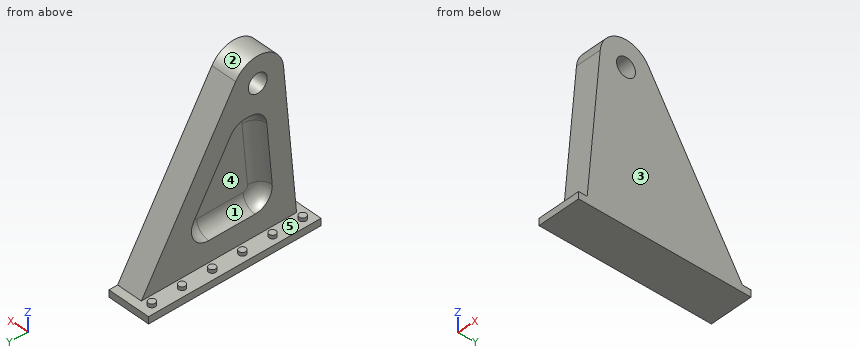
from build123d import *

# Parameters (mm, degrees)
F0_W          = 20
F0_H          = 0.8
F1_DEPTH      = 3
F1_DEPTH_BACK = 2
F2_R          = 1.1
F3_DEPTH      = 3
F5_DEPTH      = 1.5
F6_R          = 2
F7_R          = 1.49999
F8_R          = 0.4
F9_DEPTH      = 0.4


# Not quite as in the source:
# - a fillet or chamfer is up to 0.001 mm smaller than in the source, because OpenCascade refuses the exact size


with BuildPart() as f1:
    # F0 (on Right) → F1 (new body, two sides)
    with BuildSketch(Plane.YZ) as f1_sk:
        with Locations((4.5, 0.4)):
            Rectangle(F0_W, F0_H)
    extrude(amount=F1_DEPTH)
    extrude(f1_sk.sketch, amount=-F1_DEPTH_BACK)

    # F2 (on Right) → F3 (join)
    with BuildSketch(Plane.YZ):
        with BuildLine():
            Line((-4.5, 0.8), (13.5, 0.8))
            Line((13.5, 0.8), (2.5660948526, 18.8540776067))
            ThreePointArc((2.5660948526, 18.8540776067), (-0.6760626552, 20.2228306975), (-2.9878775484, 17.5694211496))
            Line((-2.9878775484, 17.5694211496), (-4.5, 0.8))
        make_face()
        with Locations((0, 17.3)):
            Circle(F2_R, mode=Mode.SUBTRACT)
    extrude(amount=F3_DEPTH)

    # F4 (on face) → F5 (cut)
    with BuildSketch(Plane(origin=(0, 0, 0), x_dir=(0, -1, 0), z_dir=(-1, 0, 0))):
        Polygon((-9.2406928099, 3.2), (1.8738512935, 3.2), (0.8819657168, 14.2), (-2.5788760591, 14.2), align=None)
    extrude(amount=-F5_DEPTH, mode=Mode.SUBTRACT)

    # F6
    f6_edges = [f1.edges().sort_by_distance(p)[0] for p in [
        (0.75, -0.881966, 14.2),
        (0.75, 2.578876, 14.2),
        (0.75, 9.240693, 3.2),
        (0.75, -1.873851, 3.2),
    ]]
    fillet(f6_edges, radius=F6_R)

    # F7 (radius 1.5 in the source; OpenCascade refuses exactly that, so slightly less here)
    f7_edges = [f1.edges().sort_by_distance(p)[0] for p in [
        (1.5, 3.002938, 3.2),
        (1.5, 7.433697, 4.218191),
        (1.5, -1.161746, 3.850783),
        (1.5, 5.282331, 9.736052),
        (1.5, -1.361712, 8.879614),
        (1.5, 2.433741, 13.942427),
        (1.5, -0.403411, 13.676352),
        (1.5, 1.198869, 14.2),
    ]]
    fillet(f7_edges, radius=F7_R)

    # F8 (on face) → F9 (join)
    with BuildSketch(Plane.XY.offset(0.8)):
        with Locations((-1, -4.3)):
            Circle(F8_R)
        with Locations((-1, -0.8)):
            Circle(F8_R)
        with Locations((-1, 2.7)):
            Circle(F8_R)
        with Locations((-1, 6.2)):
            Circle(F8_R)
        with Locations((-1, 9.7)):
            Circle(F8_R)
        with Locations((-1, 13.2)):
            Circle(F8_R)
    extrude(amount=F9_DEPTH)


solid = f1.part
Verification items for the finished model (mm, model axes). Face numbers are marked on the shaded views. A direction names the side the tool comes from. Round coordinates to 2 decimals unless told otherwise and drop trailing zeros. Loops run counter-clockwise (first coordinate to the right, second up) from the corner with the lowest first, then second, coordinate; pieces in that order, holes last. Notation, with made-up numbers: (16.25, -1) - (27.25, -1) arc R29 cw to (27.25, 22) - close; hole circle Ø1 at (-3, 2.5). An arc over 180 degrees is marked (long way). Answer in a Markdown table with one row per item. Add a question column.
Q1. Material ranges on line 1 (Z direction, x = 2.2, y = 0); line 2 (Z direction, x = -0.85, y = 2); line 3 (X direction, y = 3.75, z = 6.25), recorded low to high.
Q2. Release check for a two-part mould opening along Z. For the marked faces 3, 4 and 5 record: pulls with the +Z half, pulls with the -Z half, needs draft (parallel to the pull), parting line crosses it, or undercut.
Q3. Section check A-A on z = 17.3. Enter the section's corners in (x, y).
Q4. Gauge pin test, flat ends, axial feed: pin 1 (1.5 mm diameter, centred on x = 0.5, y = 2, fed in from +Z); pin 2 (0.9 mm diameter, centred on x = -1, y = -4.5, fed in from +Z); pin 3 (5 mm diameter, centred on y = 3, z = 10.5, fed in from -X). Record the tip position at first contact, or that the pin passes through.
Q5. Section check D-D on y = 11.5. Enter the section's corners in (x, z).
Q6. Tool access check on the marked faces 1 and 2. Record the directions out of +Z, -Z, +X, -X, +Y, -Y that give a thin tool (end or side, any length) a straight path to the whole face; none if there is none.
Q7. Section check B-B on x = 2.35. Enter the section's corners in (y, z), plus the area to 3 significant figures.
Q8. Section check C-C on y = -2.5. Enter the section's corners in (x, z), plus the area to 3 significant figures.
Found:
| question | item | result |
|---|---|---|
| 1 | line 1 | z = 0 to 16.2, 18.4 to 20.3 |
| 1 | line 2 | z = 0 to 0.8 |
| 1 | line 3 | x = 1.5 to 3 |
| 2 | face 3 | needs draft |
| 2 | face 4 | undercut |
| 2 | face 5 | pulls with the +Z half |
| 3 | outline | (0, -3.01) - (3, -3.01) - (3, -1.1) - (0, -1.1) - close; (0, 1.1) - (3, 1.1) - (3, 3.51) - (0, 3.51) - close |
| 4 | pin 1 | stops at z = 20.03 |
| 4 | pin 2 | stops at z = 1.2 |
| 4 | pin 3 | stops at x = 0 |
| 5 | outline | (-2, 0) - (3, 0) - (3, 4.1) - (0, 4.1) - (0, 0.8) - (-2, 0.8) - close |
| 6 | face 1 | -X |
| 6 | face 2 | +Z, +X, -X |
| 7 | outline | (-5.5, 0) - (14.5, 0) - (14.5, 0.8) - (13.5, 0.8) - (2.57, 18.85) arc R3 ccw to (-2.99, 17.57) - (-4.5, 0.8) - (-5.5, 0.8) - close; hole circle Ø2.2 at (0, 17.3) |
| 7 | area | 229 mm² |
| 8 | outline | (-2, 0) - (3, 0) - (3, 18.96) - (0, 18.96) - (0, 0.8) - (-2, 0.8) - close |
| 8 | area | 58.5 mm² |
